For this review, use the dimensioned drawing (mm, ordinates from the lowest corner) and the shaded views. A direction names the side the tool comes from. Coordinates: 2 decimals unless noted, no trailing zeros. Order: outer loops, then holes, each group sorted by start corner. A loop starts at its lowest first (then second) coordinate and runs counter-clockwise, first axis right, second up. Notation, with made-up numbers: M 12,53.5 L 35,53.5 A19 ccw 35,73.5 Z; hole C 52.5,79 d10. An arc over 180 degrees is marked long. Use CSV: the item, a comma, the result in double quotes.
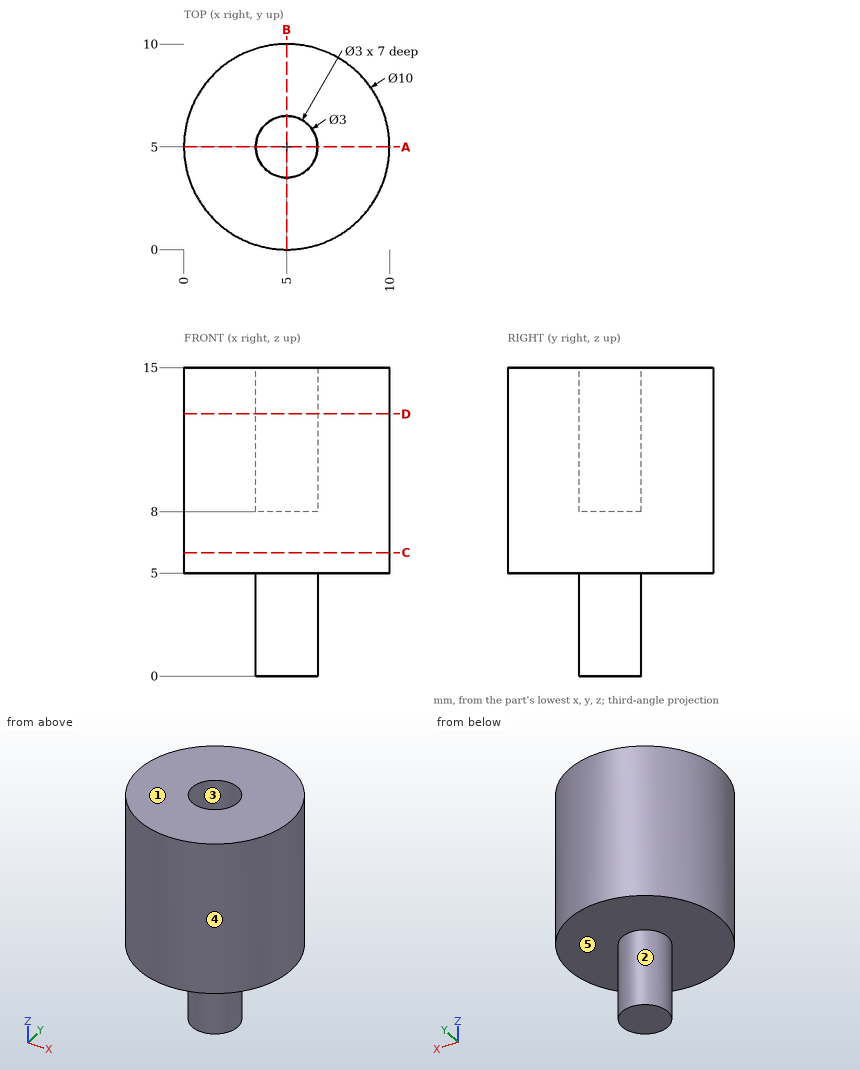
Item 1: For the marked faces 1 and 2, list the 3-axis set-ups (+Z, -Z, +X, -X, +Y, -Y) from which the entire face can be reached by the end or side of a thin tool; tool diameter is ignored.
Solutions:
face 1,"+Z, +X, -X, +Y, -Y"
face 2,"-Z"
Item 2: Add section A-A on y = 5. State the section outline as (x, z) points, and give its area (3 significant figures).
Solutions:
outline,"M 0,5 L 3.5,5 L 3.5,0 L 6.5,0 L 6.5,5 L 10,5 L 10,15 L 6.5,15 L 6.5,8 L 3.5,8 L 3.5,15 L 0,15 Z"
area,"94.0 mm^2"
Item 3: Clearance check with flat-ended pins moving along their axes: pin 1 Ø6 at (x, y) = (1, 8.5) entering from -Z; pin 2 Ø3 at (x, z) = (7.5, 9.5) entering from +Y; pin 3 Ø2 at (y, z) = (4.5, 1.5) entering from -X; pin 4 Ø2 at (x, z) = (8, 3.5) entering from +Y (3 decimals). State where each tip first meets the part, or that it passes through.
Solutions:
pin 1,"z = 5"
pin 2,"y = 9.9"
pin 3,"x = 3.5"
pin 4,"through"
Item 4: Add section C-C on z = 6. State the section outline as (x, y) points, and give its area (3 significant figures).
Solutions:
outline,"C 5,5 d10"
area,"78.5 mm^2"
Item 5: To check wall thickness, follow line 1 along Y through (x, z) = (5, 12.25); line 2 along Z through (x, y) = (7.75, 3); line 3 along X through (y, z) = (5.75, 9.75). State the ranges of each line that lie inside material, in increasing order. Write a range as [from, to].
Solutions:
line 1,"[0, 3.5], [6.5, 10]"
line 2,"[5, 15]"
line 3,"[0.06, 3.7], [6.3, 9.94]"
Item 6: Draft analysis for pull direction Y (two halves, no side actions). For the marked faces 3, 4 and 5, state which applies: released by +Y, released by -Y, zero draft, split by the parting line, or undercut.
Solutions:
face 3,"undercut"
face 4,"split by the parting line"
face 5,"zero draft"
Item 7: Add section D-D on z = 12.75. State the section outline as (x, y) points, and give its area (3 significant figures).
Solutions:
outline,"C 5,5 d10; hole C 5,5 d3"
area,"71.5 mm^2"
